Geometry check sheet. Reference: the model listing, model coordinates, mm. Give positions to 0.01 mm unless a question says otherwise; leave off trailing zeros. Write each loop counter-clockwise with the first axis right and the second up, starting at its lowest first coordinate (ties: lowest second). Pieces come first, ordered by that corner, then holes. Notation, with made-up numbers: (-36, -14.75) - (-19, -14.75) arc R8 ccw to (-19, -4.75) - close; hole circle Ø5 at (-18.75, -10). An arc over 180 degrees is marked (long way). One line per question, with ' | ' between items. Start each with the question number.
Q1. Section check B-B on x = 28. Record the boundary of the cut face in (y, z).
Q2. Gauge pin test, flat ends, axial feed: P1, Ø1, axis at y = -5, z = 1, coming from the -X side; P2, Ø1, axis at y = 1, z = 3.5, coming from the +X side. Record the tip position at first contact, or that the pin passes through.
Q3. Release check for a two-part mould opening along X. For faces 1 (the face through (-1, 0, 4)), 2 (the face through (72.15, 6.99, 1.01)), 3 (the face through (-62.07, -0.65, 2.03)), 4 (the face through (-72.15, -6.99, 1.01)) record: +X half, -X half, draft (parallel to the pull), parting line (faces both ways), or undercut.
Q4. Thickness scan on L1, parallel to X at y = 2, z = 3.65; L2, parallel to X at y = 0, z = 0.9; L3, parallel to Y at x = -65, z = 1. Record the ranges inside material, lowest first. Write a range as [from, to].
Q5. Section check A-A on z = 2.95. Count the separate pieces of the cut face and the enclosed holes in it, and give its area (3 significant figures).
Autodesk Inventor part; units mm, degrees
ref_plane "YZ Plane" through (0, 0, 0) normal (1, 0, 0) x (0, 1, 0)
ref_plane "XZ Plane" through (0, 0, 0) normal (0, 1, 0) x (-1, 0, 0)
ref_plane "XY Plane" through (0, 0, 0) normal (0, 0, 1) x (1, 0, 0)
sketch "スケッチ1" plane through (0, 0, 0) normal (0, 0, 1) x (1, 0, 0)
  line L0 (-75, 10) -> (75, 10)
  line L1 (75, 10) -> (75, -10)
  line L2 (75, -10) -> (-75, -10)
  line L3 (-75, -10) -> (-75, 10)
  line L4 (-75, 10) -> (75, -10) construction
  line L5 (75, 10) -> (-75, -10) construction
  point P0 (0, 0)
  dimension "d0" = 150
  dimension "d1" = 20
extrude "押し出し1" add sketch "スケッチ1" along normal blind 4
fillet "フィレット1" radius 10 4 edges at (75, 10, 2) (75, -10, 2) (-75, 10, 2) (-75, -10, 2)
fillet "フィレット2" radius 2 4 edges at (-72.0711, 7.0711, 4) (0, -10, 4) (72.0711, 7.0711, 4) (0, 10, 4)
sketch "スケッチ2" plane through (0, 0, 0) normal (0, 0, -1) x (-1, 0, 0)
  arc A0 (-65, 10) -> (-65, -10) centre (-65, 0) ccw
  arc A1 (65, -10) -> (65, 10) centre (65, 0) ccw
  point P0 (0, 0)
  dimension "d6" = 0
  dimension "d7" = 0
hole "穴1" at (65, 0, 0) at (-65, 0, 0) direction (0, 0, 1) diameter 6 end through all
properties part number "joy_mount_I"
Working result:
1) outline: (-10, 0) - (10, 0) - (10, 2) arc R2 ccw to (8, 4) - (-8, 4) arc R2 ccw to (-10, 2) - close
2) P1: stops at x = -73.93 | P2: stops at x = 74.68
3) face 1: draft | face 2: +X half | face 3: undercut | face 4: -X half
4) L1: x = [-73.91, -67.24], [-62.76, 62.76], [67.24, 73.91] | L2: x = [-75, -68], [-62, 62], [68, 75] | L3: y = [-10, -3], [3, 10]
5) separate pieces: 1 | enclosed holes: 2 | area: 2,780 mm2
